Input: part model. Units: mm. Frame: model coordinates. Face numbers are marked on the shaded views. A direction names the side the tool comes from. Round coordinates to 2 decimals unless told otherwise and drop trailing zeros. Write each loop counter-clockwise with the first axis right and the second up, starting at its lowest first coordinate (ties: lowest second). Pieces come first, ordered by that corner, then holes. Notation, with made-up numbers: M 64,12 L 87,12 A35 ccw 87,49 Z; hole C 23,-7.5 d3. An arc over 180 degrees is marked long. Answer as CSV lines item,"result". Start each with the question number.
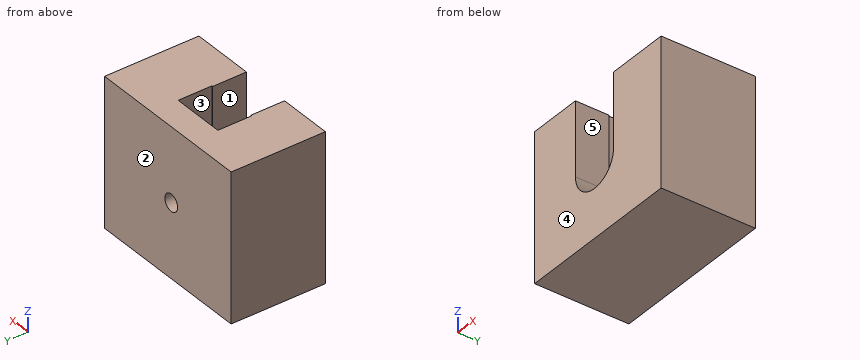
```python
from build123d import *

# Parameters (mm, degrees)
SKETCH2_W           = 200
SKETCH2_H           = 35
BOSS_EXTRUDE1_DEPTH = 30
SKETCH3_R           = 6
CUT_EXTRUDE1_DEPTH  = 203.993226488
CUT_EXTRUDE2_DEPTH  = 22
SKETCH6_W           = 22.496439662
SKETCH6_H           = 14
BOSS_EXTRUDE3_DEPTH = 38
CUT_EXTRUDE4_DEPTH  = 17.5
SKETCH9_R           = 2
CUT_EXTRUDE5_DEPTH  = 38
SKETCH10_R          = 2.25
CUT_EXTRUDE6_DEPTH  = 20
SKETCH12_W          = 4.5
SKETCH12_H          = 7.5
CUT_EXTRUDE7_DEPTH  = 46
SKETCH14_W          = 405.367486884
SKETCH14_H          = 144.136743288
CUT_EXTRUDE9_DEPTH  = 206.243757518


with BuildPart() as part:
    # Sketch2 → Boss-Extrude1 (new body)
    with BuildSketch(Plane(origin=(0, 0, 0), x_dir=(1, 0, 0), z_dir=(0, 1, 0))):
        with Locations((-100, 0)):
            Rectangle(SKETCH2_W, SKETCH2_H)
    extrude(amount=BOSS_EXTRUDE1_DEPTH)

    # Sketch3 → Cut-Extrude1 (cut, through all)
    with BuildSketch(Plane.XZ):
        with Locations(Location((-21, 0, 0), (0, 0, 270))):
            Circle(SKETCH3_R)
    extrude(amount=-CUT_EXTRUDE1_DEPTH, mode=Mode.SUBTRACT)

    # Sketch4 → Cut-Extrude2 (cut)
    with BuildSketch(Plane(origin=(0, 30, 0), x_dir=(1, 0, 0), z_dir=(0, 1, 0))):
        Polygon((-14.75, 3.608439182), (-21, 7.216878365), (-27.25, 3.608439182), (-27.25, -3.608439182), (-21, -7.216878365), (-14.75, -3.608439182), align=None)
    extrude(amount=-CUT_EXTRUDE2_DEPTH, mode=Mode.SUBTRACT)

    # Sketch6 → Boss-Extrude3 (add)
    with BuildSketch(Plane(origin=(0, 0, 0), x_dir=(0, 0, -1), z_dir=(1, 0, 0))):
        with Locations((0.204742288, 23)):
            Rectangle(SKETCH6_W, SKETCH6_H)
    extrude(amount=-BOSS_EXTRUDE3_DEPTH)

    # Sketch7 → Cut-Extrude4 (cut)
    with BuildSketch(Plane.XY.offset(17.5)):
        Polygon((-21, 16), (-14.75, 16), (-14.75, 8), (-15, 8), (-15, 0), (-27, 0), (-27, 8), (-27.25, 8), (-27.25, 16), align=None)
    extrude(amount=-CUT_EXTRUDE4_DEPTH, mode=Mode.SUBTRACT)

    # Sketch9 → Cut-Extrude5 (cut)
    with BuildSketch(Plane(origin=(0, 30, 0), x_dir=(1, 0, 0), z_dir=(0, 1, 0))):
        with Locations(Location((-21, 0, 0), (0, 0, 270))):
            Circle(SKETCH9_R)
    extrude(amount=-CUT_EXTRUDE5_DEPTH, mode=Mode.SUBTRACT)

    # Sketch10 → Cut-Extrude6 (cut)
    with BuildSketch(Plane.ZY.offset(200)):
        with Locations((6.5, 21.5)):
            Circle(SKETCH10_R)
        with Locations((6.5, 8.5)):
            Circle(SKETCH10_R)
        with Locations((-6.5, 8.5)):
            Circle(SKETCH10_R)
        with Locations((-6.5, 21.5)):
            Circle(SKETCH10_R)
    extrude(amount=-CUT_EXTRUDE6_DEPTH, mode=Mode.SUBTRACT)

    # Sketch12 → Cut-Extrude7 (cut)
    with BuildSketch(Plane(origin=(0, 30, 0), x_dir=(1, 0, 0), z_dir=(0, 1, 0))):
        with Locations((-191.75, -6.5625)):
            Rectangle(SKETCH12_W, SKETCH12_H)
        with Locations((-191.75, 6.5625)):
            Rectangle(SKETCH12_W, SKETCH12_H)
    extrude(amount=-CUT_EXTRUDE7_DEPTH, mode=Mode.SUBTRACT)

    # Sketch14 → Cut-Extrude9 (cut, through all)
    # profile 1 of 2: a face of its own
    with BuildSketch(Plane.XY.offset(17.5)):
        with Locations((-15, 0)):
            Rectangle(SKETCH14_W, SKETCH14_H)
        Polygon((0, 30), (0, 22.340454029), (9.526767724, 22.340454029), (9.526767724, -15.531579882), (-39.86578, -15.531579882), (-39.86578, 0), (-200, 0), (-200, 30), align=None, mode=Mode.SUBTRACT)
    # profile 2 of 2: a face of its own
    with BuildSketch(Plane.XY.offset(17.5)):
        Polygon((-39.86578, 0), (-39.86578, 22.340454029), (0, 22.340454029), (0, 30), (-200, 30), (-200, 0), align=None)
    extrude(amount=-CUT_EXTRUDE9_DEPTH, mode=Mode.SUBTRACT)


solid = part.part
```
Item 1: Access query for the marked faces 4 and 5. Directions: +Z, -Z, +X, -X, +Y, -Y. A direction counts if a zero-diameter tool reaches every point of the face in a straight line with its end or side. Return the directions, or none.
Item 2: Cut plane B-B, the plane z = 11.5. Return loops of the section in (x, y), plus the area to 3 significant figures.
Item 3: Cut plane A-A, the plane y = 9.5. Return loops of the section in (x, z).
Item 4: Cut plane D-D, the plane z = -6.5. Return loops of the section in (x, y), plus the area to 3 significant figures.
Item 5: Cut plane C-C, the plane x = -26.5. Return loops of the section in (y, z).
Item 6: Draft query along Y for the marked faces 1, 2 and 3. Return one class per face: +Y half, -Y half, draft (parallel to the pull), parting line (faces both ways), or undercut.
Item 7: Line query: line 1 (X direction, y = 11.5, z = 12); line 2 (X direction, y = 20.25, z = 0); line 3 (Y direction, x = -23, z = -1). Output: solid intervals per line, ascending. Write a range as [from, to].
Item 8: Pin query (flat end, axial travel): pin 1 Ø12 at (y, z) = (18, -10) entering from +X; pin 2 Ø6 at (x, z) = (-21.5, 8) entering from -Y; pin 3 Ø2.5 at (x, z) = (-21, 0) entering from -Y. Return the tip coordinate at first contact, or that it passes through.
Results list:
1,face 4,"+Z, -Z, +X, -X, -Y"
1,face 5,"+Z, -Y"
2,outline,"M -39.87,0 L -27,0 L -27,8 L -27.25,8 L -27.25,16 L -14.75,16 L -14.75,8 L -15,8 L -15,0 L 0,0 L 0,22.34 L -39.87,22.34 Z"
2,area,"695 mm²"
3,outline,"M -39.87,-17.5 L 0,-17.5 L 0,17.5 L -14.75,17.5 L -14.75,-3.61 L -21,-7.22 L -27.25,-3.61 L -27.25,17.5 L -39.87,17.5 Z"
4,outline,"M -39.87,0 L 0,0 L 0,22.34 L -39.87,22.34 Z; hole M -22.24,8 L -19.76,8 L -19.76,16 L -22.24,16 Z"
4,area,"871 mm²"
5,outline,"M 0,-17.5 L 22.34,-17.5 L 22.34,17.5 L 16,17.5 L 16,-4.04 L 8,-4.04 L 8,-2.4 L 0,-2.4 Z"
6,face 1,"draft"
6,face 2,"+Y half"
6,face 3,"undercut"
7,line 1,"[-39.87, -27.25], [-14.75, 0]"
7,line 2,"[-39.87, -23], [-19, 0]"
7,line 3,"[16, 22.34]"
8,pin 1,"x = 0"
8,pin 2,"y = 16"
8,pin 3,"through"
